Can you work these out from the model? Positions are in its coordinate system, mm. A direction names the side the tool comes from. Coordinates: 2 decimals unless noted, no trailing zeros. Write each loop counter-clockwise with the first axis right and the second up, starting at its lowest first coordinate (ties: lowest second). Pieces come first, ordered by that corner, then holes. Notation, with made-up numbers: M -6.75,78.25 L -0.75,78.25 A10 cw -0.75,94.25 Z; hole C 18,-19 d9. An arc over 180 degrees is marked long. Answer as a JSON object with one key per item and string values. Group by question number.
from build123d import *

# Parameters (mm, degrees)
SKETCH_W        = 160
SKETCH_H        = 57
SKETCH_W_2      = 156
SKETCH_H_2      = 53
PAD_DEPTH       = 23.1
SKETCH001_W     = 160
SKETCH001_H     = 57
PAD001_DEPTH    = 1
SKETCH002_R     = 10.75
SKETCH002_R_2   = 2.97
SKETCH002_R_3   = 1.6
SKETCH002_W     = 101.49
SKETCH002_H     = 36.46
POCKET_DEPTH    = 1
SKETCH003_W     = 6
SKETCH003_H     = 2.1
SKETCH003_W_2   = 14
SKETCH003_H_2   = 12
POCKET001_DEPTH = 5
SKETCH005_W     = 57
SKETCH005_H     = 2
PAD002_DEPTH    = 2


with BuildPart() as part:
    # Sketch → Pad (new body)
    with BuildSketch(Plane.XY):
        with Locations((8.261541, -8.185916)):
            Rectangle(SKETCH_W, SKETCH_H)
        with Locations((8.261541, -8.185916)):
            Rectangle(SKETCH_W_2, SKETCH_H_2, mode=Mode.SUBTRACT)
    extrude(amount=PAD_DEPTH)

    # Sketch001 → Pad001 (new body)
    with BuildSketch(Plane.XY.offset(23.1)):
        with Locations((8.261541, -8.185916)):
            Rectangle(SKETCH001_W, SKETCH001_H)
    extrude(amount=PAD001_DEPTH)

    # Sketch002 → Pocket (cut)
    with BuildSketch(Plane.XY.offset(24.1)):
        with Locations((71.821541, -6.710916)):
            Circle(SKETCH002_R)
        with Locations((50.211541, -20.210916)):
            Circle(SKETCH002_R_2)
        with Locations((50.211541, 7.179084)):
            Circle(SKETCH002_R_2)
        with Locations((50.211541, -7.130916)):
            Circle(SKETCH002_R_3)
        with Locations((-14.493459, -6.515916)):
            Rectangle(SKETCH002_W, SKETCH002_H)
    extrude(amount=-POCKET_DEPTH, mode=Mode.SUBTRACT)

    # Sketch003 → Pocket001 (cut)
    with BuildSketch(Plane(origin=(-71.738459, 0, 0), x_dir=(0, -1, 0), z_dir=(-1, 0, 0))):
        with Locations((-13.314084, 1.05)):
            Rectangle(SKETCH003_W, SKETCH003_H)
        with Locations((6.700916, 12.6)):
            Rectangle(SKETCH003_W_2, SKETCH003_H_2)
        with Locations((29.685916, 1.05)):
            Rectangle(SKETCH003_W, SKETCH003_H)
    extrude(amount=-POCKET001_DEPTH, mode=Mode.SUBTRACT)

    # Sketch005 → Pad002 (new body)
    with BuildSketch(Plane(origin=(-71.738459, 0, 0), x_dir=(0, -1, 0), z_dir=(-1, 0, 0))):
        with Locations((8.185916, -1)):
            Rectangle(SKETCH005_W, SKETCH005_H)
    extrude(amount=-PAD002_DEPTH)


solid = part.part
Q1. If we section it at C-C on z = 9.5: List the corners of the cut face in (x, y) for me.
Q2. On a 3-axis mill with a long thin cutter (end or side, diameter ignored), from which of +Z, -Z, +X, -X, +Y, -Y can I reach the whole of each face in a straight line? I mean faces 5 (the flat face through (25, -27, 24.1)), 6 (the flat face through (-69.738, -8, 5)), 7 (the flat face through (9, 19, 0)). Say none if no direction works.
Q3. We'd pull the mould along Y, two halves only. Please class faces 1 (the flat face through (88.262, -9, 12)), 2 (the flat face through (7, 18.314, 11)), 3 (the flat face through (7, -36.686, 14)), 4 (the flat face through (7, 20.314, 14)): pulls with the +Y half, pulls with the -Y half, needs draft (parallel to the pull), parting line crosses it, or undercut.
Q4. If we section it at B-B on y = 14.5: List the corners of the cut face in (x, z) for me.
Q5. Will this pin go through, and if not, where does the flat tip stop? pin 1 (12 mm diameter, centred on x = 12, y = 13.5, fed in from -Z).
Q6. Please list where these lines run through material, in increasing order: L1, parallel to Y at x = 63.5, z = 16.25; L2, parallel to X at y = -31.5, z = 4.25; L3, parallel to X at y = -4, z = 13.5.
Q7. If we section it at A-A on x = -18: List the corners of the cut face in (y, z) for me.
Q8. If we section it at D-D on x = 55.5: List the corners of the cut face in (y, z) for me, and give its area (3 significant figures).
Reply:
{
 "1": {"outline": "M -71.74,-36.69 L 88.26,-36.69 L 88.26,20.31 L -71.74,20.31 L -71.74,0.3 L -69.74,0.3 L -69.74,18.31 L 86.26,18.31 L 86.26,-34.69 L -69.74,-34.69 L -69.74,-13.7 L -71.74,-13.7 Z"},
 "2": {"face 5": "+Z, +X, -X, +Y, -Y", "face 6": "-Z", "face 7": "-Z, +X, +Y, -Y"},
 "3": {"face 1": "needs draft", "face 2": "undercut", "face 3": "pulls with the -Y half", "face 4": "pulls with the +Y half"},
 "4": {"outline": "M -71.74,-2 L -69.74,-2 L -69.74,0 L -71.74,0 Z; M -71.74,2.1 L -69.74,2.1 L -69.74,23.1 L 86.26,23.1 L 86.26,0 L 88.26,0 L 88.26,24.1 L -71.74,24.1 Z"},
 "5": {"pin 1": "z = 0"},
 "6": {"L1": "-36.69 to -34.69, 18.31 to 20.31", "L2": "-71.74 to -69.74, 86.26 to 88.26", "L3": "86.26 to 88.26"},
 "7": {"outline": "M -36.69,0 L -34.69,0 L -34.69,23.1 L -24.75,23.1 L -24.75,24.1 L -36.69,24.1 Z; M 11.71,23.1 L 18.31,23.1 L 18.31,0 L 20.31,0 L 20.31,24.1 L 11.71,24.1 Z"},
 "8": {"outline": "M -36.69,0 L -34.69,0 L -34.69,23.1 L 18.31,23.1 L 18.31,0 L 20.31,0 L 20.31,24.1 L -36.69,24.1 Z", "area": "149 mm^2"}
}
